Autodesk Inventor part; units mm, degrees
ref_plane "Work Plane1" through (0, 17.625, 0) normal (0, 1, 0) x (-1, 0, 0)
ref_plane "Work Plane2" through (0, 14.1, 0) normal (0, 1, 0) x (-1, 0, 0)
ref_plane "YZ Plane" through (0, 0, 0) normal (1, 0, 0) x (0, 1, 0)
sketch "Sketch1" plane through (0, 0, 0) normal (0, 0, 1) x (1, 0, 0)
  circle A0 centre (0, 0) radius 17.25
  circle A1 centre (0, 0) radius 17.375
  dimension "d0" = 34.5
  dimension "d1" = 34.75
extrude "Extrusion1" add sketch "Sketch1" along normal mid plane 17
sketch "Sketch2" plane through (0, 0, 0) normal (0, 0, 1) x (1, 0, 0)
  circle A0 centre (0, 0) radius 17.375
  circle A1 centre (0, 0) radius 17.625
  dimension "d4" = 34.75
  dimension "d5" = 0.25
extrude "Extrusion2" add sketch "Sketch2" along normal blind 8.75 and the other way blind 8.25
ref_plane "Work Plane1" through (0, 17.625, 0) normal (0, 1, 0) x (-1, 0, 0)
sketch "Sketch3" plane through (0, 17.625, 0) normal (0, 1, 0) x (-1, 0, 0)
  line L0 (10, 0) -> (10, -8.5)
  line L1 (10, -8.5) -> (0, -8.5)
  line L2 (-10, 0) -> (-10, 9.4902)
  line L3 (-10, 9.4902) -> (-0.099, 9.4902)
  line L4 (10, -8.5) -> (-10, -8.5)
  line L5 (-10, -8.5) -> (-10, 9.4902)
  line L6 (-10, 9.4902) -> (10, 9.4902)
  line L7 (10, 9.4902) -> (10, -8.5)
  point P0 (0, 0)
  point P1 (-0.099, 9.4902)
  dimension "d10" = 10
  dimension "d11" = 10
extrude "Extrusion3" cut sketch "Sketch3" against normal blind 8.75
ref_plane "Work Plane2" through (0, 14.1, 0) normal (0, 1, 0) x (-1, 0, 0)
sketch "Sketch4" plane through (0, 14.1, 0) normal (0, 1, 0) x (-1, 0, 0)
  line L0 (-10, -8.25) -> (-10, 8.75)
  line L1 (10, -8.25) -> (-10, -8.25)
  line L2 (-10, -8.25) -> (-10, 8.75)
  line L3 (-10, 8.75) -> (10, 8.75)
  line L4 (10, 8.75) -> (10, -8.25)
  point P0 (0, 0)
extrude "Extrusion4" add sketch "Sketch4" along normal blind 0.25
sketch "Sketch5" plane through (0, 14.35, 0) normal (0, 1, 0) x (1, 0, 0)
  line L0 (-2.4, 5.75) -> (2.4, 5.75)
  line L1 (2.4, 5.75) -> (2.4, -6.25)
  line L2 (2.4, -6.25) -> (-2.4, -6.25)
  line L3 (-2.4, -6.25) -> (-2.4, 5.75)
  line L4 (10, 8.25) -> (-10, 8.25)
  line L5 (10, 8.25) -> (10, -8.75)
  point P0 (0, 0)
  dimension "d17" = 4.8
  dimension "d18" = 12
  dimension "d19" = 2.5
  dimension "d20" = 7.6
extrude "Extrusion5" add sketch "Sketch5" along normal blind 2.4
sketch "Sketch6" plane through (2.4, 14.35, 6.25) normal (1, 0, 0) x (0, 0, -1)
  line L0 (12, 0) -> (12, 2.4)
  line L1 (12, 0) -> (9.6, 2.4)
  line L2 (12, 2.4) -> (0, 2.4)
  line L3 (12, 0) -> (15.3941, 0) construction
  line L4 (9.6, 2.4) -> (12, 2.4)
  line L5 (12, 2.4) -> (12, 0)
  point P0 (6.25, -14.35)
  dimension "d23" = 135
extrude "Extrusion6" cut sketch "Sketch6" against normal blind 4.8
properties part number "Large_Ring"
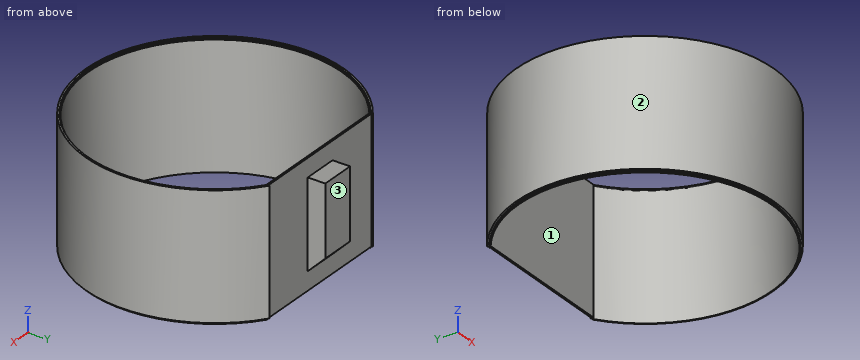
Work out the finished part from the listing and answer in its coordinate system (mm). Face numbers are marked on the shaded views. Give positions to 0.01 mm unless a question says otherwise; leave off trailing zeros. Loops run counter-clockwise (first coordinate to the right, second up) from the corner with the lowest first, then second, coordinate; pieces in that order, holes last. Notation, with made-up numbers: (-26.5, 60) -> (1.5, 60) arc R8 cw to (1.5, 65) -> close; hole circle Ø6 at (17, 52). An arc over 180 degrees is marked (long way). Use a Markdown table: item, result. Add a question column.
1) Consider line 1 along X through (y, z) = (0, -3.25) (3 decimals); line 2 along X through (y, z) = (0, 8.65) (3 decimals); line 3 along Y through (x, z) = (5, 0). Determine where each line is inside the solid, lowest interval first.
2) The part is cut by section B-B, the plane z = 7.5. Determine the outline of the cut face in (x, y) (3 decimals).
3) The part is cut by section D-D, the plane z = 1.5. Determine the outline of the cut face in (x, y) (3 decimals), plus the area to 3 significant figures.
4) The part is cut by section C-C, the plane x = 0. Determine the outline of the cut face in (y, z) (3 decimals), plus the area to 3 significant figures.
5) Each of these flat-tipped pins is pushed along its axis until it touches: P1, Ø8, axis at y = 4.5, z = -3, coming from the -X side; P2, Ø6, axis at y = 10.5, z = 6, coming from the +X side; P3, Ø1.9, axis at y = 15, z = 0, coming from the -X side. Where does it stop, or does it pass through?
6) For a pull along X with two mould halves and no side action, classify the marked faces 1, 2 and 3 as +X half, -X half, draft (parallel to the pull), parting line (faces both ways), or undercut.
Reported:
| question | item | result |
|---|---|---|
| 1 | line 1 | x = -17.625 to -17.25, 17.25 to 17.625 |
| 1 | line 2 | x = -17.625 to -17.375, 17.375 to 17.625 |
| 1 | line 3 | y = -16.9 to -16.51, 14.1 to 14.35 |
| 2 | outline | (-10, 14.35) -> (-10, 14.513) arc R17.625 ccw (long way) to (10, 14.513) -> (10, 14.35) -> close; hole (-10, 14.056) arc R17.25 ccw (long way) to (10, 14.056) -> (10, 14.1) -> (-10, 14.1) -> close |
| 3 | outline | (-10, 14.35) -> (-10, 14.513) arc R17.625 ccw (long way) to (10, 14.513) -> (10, 14.35) -> (2.4, 14.35) -> (2.4, 16.75) -> (-2.4, 16.75) -> (-2.4, 14.35) -> close; hole (-10, 14.056) arc R17.25 ccw (long way) to (10, 14.056) -> (10, 14.1) -> (-10, 14.1) -> close |
| 3 | area | 49.6 mm^2 |
| 4 | outline | (-17.625, -8.25) -> (-17.375, -8.25) -> (-17.375, -8.5) -> (-17.25, -8.5) -> (-17.25, 8.5) -> (-17.375, 8.5) -> (-17.375, 8.75) -> (-17.625, 8.75) -> close; (14.1, -8.25) -> (14.35, -8.25) -> (14.35, -5.75) -> (16.75, -3.35) -> (16.75, 6.25) -> (14.35, 6.25) -> (14.35, 8.75) -> (14.1, 8.75) -> close |
| 4 | area | 36.5 mm^2 |
| 5 | P1 | stops at x = -17.62 |
| 5 | P2 | stops at x = 15.95 |
| 5 | P3 | stops at x = -10.64 |
| 6 | face 1 | undercut |
| 6 | face 2 | parting line |
| 6 | face 3 | draft |
